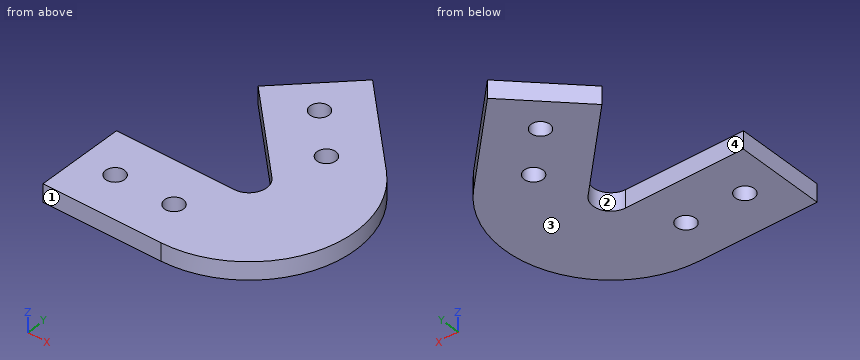
from build123d import *

# Parameters (mm, degrees)
SKETCH_1_W          = 20
SKETCH_1_H          = 15
EXTRUDE_1_DEPTH     = 3
SKETCH_2_R          = 1.6
CUT_EXTRUDE_1_DEPTH = 3


with BuildPart() as part:
    # 草图1 → 凸台-拉伸1 (new body)
    with BuildSketch(Plane.XY):
        Polygon((62.111299198, 206.50315886), (76.253434822, 192.361023236), (86.86003654, 202.967624954), (72.717900916, 217.109760578), align=None)
        with BuildLine():
            ThreePointArc((86.86003654, 202.967624954), (90.761946064, 183.35140111), (74.132114478, 172.239702893))
            Line((74.132114478, 172.239702893), (74.132114478, 187.239702893))
            ThreePointArc((74.132114478, 187.239702893), (76.903753076, 189.091652596), (76.253434822, 192.361023236))
            Line((76.253434822, 192.361023236), (86.86003654, 202.967624954))
        make_face()
        with Locations((64.132114478, 179.739702893)):
            Rectangle(SKETCH_1_W, SKETCH_1_H)
    extrude(amount=EXTRUDE_1_DEPTH)

    # 草图2 → 切除-拉伸1 (cut)
    with BuildSketch(Plane.XY.offset(3)):
        with Locations((71.657240744, 207.563819032)):
            Circle(SKETCH_2_R)
        with Locations((78.728308556, 200.49275122)):
            Circle(SKETCH_2_R)
        with Locations((60.132114478, 179.739702893)):
            Circle(SKETCH_2_R)
        with Locations((70.132114478, 179.739702893)):
            Circle(SKETCH_2_R)
    extrude(amount=-CUT_EXTRUDE_1_DEPTH, mode=Mode.SUBTRACT)


solid = part.part
Can you work these out from the model? Positions are in its coordinate system, mm. Face numbers are marked on the shaded views. Coordinates: 2 decimals unless noted, no trailing zeros. Write each loop counter-clockwise with the first axis right and the second up, starting at its lowest first coordinate (ties: lowest second). Pieces come first, ordered by that corner, then holes. Notation, with made-up numbers: (-22, 34.5) -> (-3, 34.5) arc R17 ccw to (-3, 60.5) -> close; hole circle Ø1 at (7, 26.25). An arc over 180 degrees is marked (long way). Write item = value, one per line.
(1) Imagine slicing it at C-C (z = 1.1). Please give me the cut outline in (x, y).
Verdict:
outline = (54.13, 172.24) -> (74.13, 172.24) arc R18 ccw to (86.86, 202.97) -> (72.72, 217.11) -> (62.11, 206.5) -> (76.25, 192.36) arc R3 cw to (74.13, 187.24) -> (54.13, 187.24) -> close; hole circle Ø3.2 at (60.13, 179.74); hole circle Ø3.2 at (70.13, 179.74); hole circle Ø3.2 at (71.66, 207.56); hole circle Ø3.2 at (78.73, 200.49)
(2) Thinking about a two-plate mould opening in Y: for the marked faces 1, 2, 3 and 4, which applies, +Y half, -Y half, draft (parallel to the pull), parting line (faces both ways), or undercut?
Verdict:
face_1 = -Y half
face_2 = undercut
face_3 = draft
face_4 = undercut
(3) Imagine slicing it at B-B (x = 71). Please give me the cut outline in (y, z), and give its area (3 significant figures).
Verdict:
outline = (172.24, 0) -> (178.4, 0) -> (178.4, 3) -> (172.24, 3) -> close; (181.08, 0) -> (187.24, 0) -> (187.24, 3) -> (181.08, 3) -> close; (197.61, 0) -> (206.11, 0) -> (206.11, 3) -> (197.61, 3) -> close; (209.02, 0) -> (215.39, 0) -> (215.39, 3) -> (209.02, 3) -> close
area = 81.5 mm^2
(4) Imagine slicing it at A-A (x = 59.5). Please give me the cut outline in (y, z), and give its area (3 significant figures).
Verdict:
outline = (172.24, 0) -> (178.27, 0) -> (178.27, 3) -> (172.24, 3) -> close; (181.21, 0) -> (187.24, 0) -> (187.24, 3) -> (181.21, 3) -> close
area = 36.2 mm^2
(5) Imagine slicing it at D-D (y = 210). Please give me the cut outline in (x, z), and give its area (3 significant figures).
Verdict:
outline = (65.61, 0) -> (79.83, 0) -> (79.83, 3) -> (65.61, 3) -> close
area = 42.7 mm^2
(6) For pin 1 (0.9 mm diameter, centred on x = 64, z = 2, fed in from +Y); pin 2 (1.5 mm diameter, centred on x = 59, z = 1.5, fed in from +Y), each with a flat end and sliding along its axis, tell me the tip position at first contact or that it passes through.
Verdict:
pin_1 = 208.84
pin_2 = 187.24
(7) If I drill on probe 1 along X at (y, z) = (179.5, 2.05); probe 2 along Y at (x, z) = (73, 1.35); probe 3 along Y at (x, z) = (78, 1.5), over which ranges is the centre line in solid material (lowest first)?
Verdict:
probe_1 = 54.13 to 58.55, 61.71 to 68.55, 71.71 to 88.58
probe_2 = 172.24 to 187.24, 195.61 to 206.69, 208.43 to 216.83
probe_3 = 172.66 to 199.07, 201.92 to 211.83
